```python
from build123d import *

# Parameters (mm, degrees)
SKETCH1_R           = 1.55
SKETCH1_R_2         = 2.25
BOSS_EXTRUDE1_DEPTH = 6
SKETCH4_W           = 6
SKETCH4_H           = 15
BOSS_EXTRUDE3_DEPTH = 4.64


with BuildPart() as part:
    # Sketch1 → Boss-Extrude1 (new body)
    with BuildSketch(Plane.XY):
        with BuildLine():
            Line((5, 0), (70, 0))
            ThreePointArc((70, 0), (73.535533906, -1.464466094), (75, -5))
            Line((75, -5), (75, -20))
            ThreePointArc((75, -20), (73.535533906, -23.535533906), (70, -25))
            Line((70, -25), (5, -25))
            ThreePointArc((5, -25), (1.464466094, -23.535533906), (0, -20))
            Line((0, -20), (0, -5))
            ThreePointArc((0, -5), (1.464466094, -1.464466094), (5, 0))
        make_face()
        with Locations((7, -7)):
            Circle(SKETCH1_R, mode=Mode.SUBTRACT)
        with Locations((7, -18)):
            Circle(SKETCH1_R, mode=Mode.SUBTRACT)
        with Locations((68, -7)):
            Circle(SKETCH1_R, mode=Mode.SUBTRACT)
        with Locations((68, -18)):
            Circle(SKETCH1_R, mode=Mode.SUBTRACT)
        with Locations((19, -5.5)):
            Circle(SKETCH1_R_2, mode=Mode.SUBTRACT)
        with Locations((19, -19.5)):
            Circle(SKETCH1_R_2, mode=Mode.SUBTRACT)
        with Locations((56, -5.5)):
            Circle(SKETCH1_R_2, mode=Mode.SUBTRACT)
        with Locations((56, -19.5)):
            Circle(SKETCH1_R_2, mode=Mode.SUBTRACT)
    extrude(amount=BOSS_EXTRUDE1_DEPTH)

    # Sketch4 → Boss-Extrude3 (add)
    with BuildSketch(Plane(origin=(75, 0, 0), x_dir=(0, 0, -1), z_dir=(1, 0, 0))):
        with Locations((-3, -12.5)):
            Rectangle(SKETCH4_W, SKETCH4_H)
    extrude(amount=BOSS_EXTRUDE3_DEPTH)


solid = part.part
```
Verification items for the finished model (mm, model axes). A direction names the side the tool comes from. Round coordinates to 2 decimals unless told otherwise and drop trailing zeros. Order: outer loops, then holes, each group sorted by start corner. A loop starts at its lowest first (then second) coordinate and runs counter-clockwise, first axis right, second up. Notation, with made-up numbers: (33, -14.5) -> (73, -14.5) arc R11 ccw to (73, -5.5) -> close; hole circle Ø8 at (82.5, 39). An arc over 180 degrees is marked (long way). Put each result on its own line as item: value. Start each with the question number.
(1) Draft check along Y on faces 1 (the face through (77, -5, 3)), 2 (the face through (79.64, -12, 3)), 3 (the face through (69.478, -17.534, 2.958)), 4 (the face through (2, -24, 3)). Enter one of: +Y half, -Y half, draft (parallel to the pull), parting line (faces both ways), or undercut.
(2) Material ranges on line 1 along Y through (x, z) = (56, 2.8); line 2 along Y through (x, z) = (7, 3.5); line 3 along X through (y, z) = (-21.25, 1.35), recorded low to high.
(3) Section check A-A (x = 68). Enter the section's corners in (y, z), then the cut area to 3 significant figures.
(4) Tool access check on faces 5 (the face through (54.214, -20.869, 2.958)), 6 (the face through (77, -20, 3)). Record the directions out of +Z, -Z, +X, -X, +Y, -Y that give a thin tool (end or side, any length) a straight path to the whole face; none if there is none.
(5) Section check C-C (z = 4.1). State how many separate pieces and enclosed holes the cut face has, then the cut area to 3 significant figures.
(6) Section check D-D (y = -2.25). Enter the section's corners in (x, z).
(7) Depth check by flat-ended pin: pin 1 Ø3.5 at (x, z) = (76, 2.5) entering from +Y. Enter the tip coordinate at first touch or a pass-through.
(8) Section check B-B (y = -21). Enter the section's corners in (x, z), then the cut area to 3 significant figures.
Completed:
1. face 1: +Y half
1. face 2: draft
1. face 3: undercut
1. face 4: -Y half
2. line 1: y = -25 to -21.75, -17.25 to -7.75, -3.25 to 0
2. line 2: y = -25 to -19.55, -16.45 to -8.55, -5.45 to 0
2. line 3: x = 0.16 to 17.59, 20.41 to 54.59, 57.41 to 74.84
3. outline: (-25, 0) -> (-19.55, 0) -> (-19.55, 6) -> (-25, 6) -> close; (-16.45, 0) -> (-8.55, 0) -> (-8.55, 6) -> (-16.45, 6) -> close; (-5.45, 0) -> (0, 0) -> (0, 6) -> (-5.45, 6) -> close
3. area: 113 mm2
4. face 5: +Z, -Z
4. face 6: +Z, -Z, +X, -Y
5. separate pieces: 1
5. enclosed holes: 8
5. area: 1,830 mm2
6. outline: (0.82, 0) -> (74.18, 0) -> (74.18, 6) -> (0.82, 6) -> close
7. pin 1: stops at y = -2.37
8. outline: (0.1, 0) -> (17.32, 0) -> (17.32, 6) -> (0.1, 6) -> close; (20.68, 0) -> (54.32, 0) -> (54.32, 6) -> (20.68, 6) -> close; (57.68, 0) -> (74.9, 0) -> (74.9, 6) -> (57.68, 6) -> close
8. area: 409 mm2
